```python
from build123d import *

# Parameters (mm, degrees)
SKIZZE1_W                       = 42.3
SKIZZE1_H                       = 47.3
SKIZZE1_R                       = 12
AUFSATZ_LINEAR_AUSTRAGEN1_DEPTH = 2
SKIZZE2_W                       = 42.3
SKIZZE2_H                       = 2
AUFSATZ_LINEAR_AUSTRAGEN2_DEPTH = 48


with BuildPart() as part:
    # Skizze1 → Aufsatz-Linear austragen1 (new body)
    with BuildSketch(Plane(origin=(0, 12.133771831, 0), x_dir=(1, 0, 0), z_dir=(0, 1, 0))):
        with Locations((-2.775765494, -2.5)):
            Rectangle(SKIZZE1_W, SKIZZE1_H)
        with Locations(Location((-2.775765494, 0, 0), (0, 0, 270))):
            Circle(SKIZZE1_R, mode=Mode.SUBTRACT)
    extrude(amount=AUFSATZ_LINEAR_AUSTRAGEN1_DEPTH)

    # Skizze2 → Aufsatz-Linear austragen2 (add)
    with BuildSketch(Plane.XZ.offset(-12.133771831)):
        with Locations((-2.775765494, 25.15)):
            Rectangle(SKIZZE2_W, SKIZZE2_H)
    extrude(amount=AUFSATZ_LINEAR_AUSTRAGEN2_DEPTH)


solid = part.part
```
Work out the finished part from the listing and answer in its coordinate system (mm). A direction names the side the tool comes from. Give positions to 0.01 mm unless a question says otherwise; leave off trailing zeros. Write each loop counter-clockwise with the first axis right and the second up, starting at its lowest first coordinate (ties: lowest second). Pieces come first, ordered by that corner, then holes. Notation, with made-up numbers: (47.25, -2.5) -> (72.25, -2.5) arc R36 ccw to (72.25, 33.5) -> close; hole circle Ø3 at (9.25, 71.25). An arc over 180 degrees is marked (long way). Write each question's results on one line, items separated by ' | '.
1. This flat-tipped pin is pushed along its axis until it touches: pin 1 Ø10 at (x, y) = (1.5, -12.5) entering from -Z. Where does it stop, or does it pass through?
Data:
pin 1: z = 24.15
2. Determine the mould class of faces 1 (the flat face through (-23.926, 0, 25)), 2 (the flat face through (-3, -35.866, 25)), 3 (the cylindrical face through (0.829, 13.12, 11.446)), 4 (the flat face through (18.374, 0, 25)) for opening direction X: +X half, -X half, draft (parallel to the pull), parting line (faces both ways), or undercut.
Data:
face 1: -X half | face 2: draft | face 3: undercut | face 4: +X half
3. Find section A-A on z = -8.5. Determine the outline of the cut face in (x, y), and give its area (3 significant figures).
Data:
outline: (-23.93, 12.13) -> (-11.25, 12.13) -> (-11.25, 14.13) -> (-23.93, 14.13) -> close; (5.69, 12.13) -> (18.37, 12.13) -> (18.37, 14.13) -> (5.69, 14.13) -> close | area: 50.7 mm^2
4. Find section D-D on x = 6. Determine the outline of the cut face in (y, z).
Data:
outline: (-35.87, 24.15) -> (12.13, 24.15) -> (12.13, 8.18) -> (14.13, 8.18) -> (14.13, 26.15) -> (-35.87, 26.15) -> close; (12.13, -21.15) -> (14.13, -21.15) -> (14.13, -8.18) -> (12.13, -8.18) -> close
5. Find section B-B on x = -9.5. Determine the outline of the cut face in (y, z).
Data:
outline: (-35.87, 24.15) -> (12.13, 24.15) -> (12.13, 9.94) -> (14.13, 9.94) -> (14.13, 26.15) -> (-35.87, 26.15) -> close; (12.13, -21.15) -> (14.13, -21.15) -> (14.13, -9.94) -> (12.13, -9.94) -> close
6. Straight lines are drawn through the part: L1, parallel to X at y = 12.9, z = 0; L2, parallel to Z at x = 0.5, y = 4; L3, parallel to Y at x = -15.5, z = -8. For each, find the intervals that lie inside material, in ascending order.
Data:
L1: -23.93 to -14.78, 9.22 to 18.37 | L2: 24.15 to 26.15 | L3: 12.13 to 14.13
7. Find section C-C on z = 0. Determine the outline of the cut face in (x, y), and give its area (3 significant figures).
Data:
outline: (-23.93, 12.13) -> (-14.78, 12.13) -> (-14.78, 14.13) -> (-23.93, 14.13) -> close; (9.22, 12.13) -> (18.37, 12.13) -> (18.37, 14.13) -> (9.22, 14.13) -> close | area: 36.6 mm^2
8. A tool of negligible diameter and unlimited length cuts with its end or side. For faces 5 (the flat face through (-3, 14.134, 13)), 6 (the flat face through (-8, 12.134, 11)), from which of +Z, -Z, +X, -X, +Y, -Y can it reach the whole face along a straight path? Write none if from no direction.
Data:
face 5: +Z, -Z, +X, -X, +Y | face 6: -Z, +X, -X, -Y
